from build123d import *

# Parameters (mm, degrees)
SKETCH1_R           = 20
SKETCH1_R_2         = 9.5
BOSS_EXTRUDE1_DEPTH = 55
SKETCH2_R           = 3.5
CUT_EXTRUDE1_DEPTH  = 12.66666667


with BuildPart() as part:
    # Sketch1 → Boss-Extrude1 (new body)
    with BuildSketch(Plane.XY):
        Circle(SKETCH1_R)
        Circle(SKETCH1_R_2, mode=Mode.SUBTRACT)
    extrude(amount=BOSS_EXTRUDE1_DEPTH)

    # Sketch2 → Cut-Extrude1 (cut, through all)
    with BuildSketch(Plane(origin=(8.33333333, 0, 0), x_dir=(0, 0, -1), z_dir=(1, 0, 0))):
        with Locations((-47.428775099, 14.493654617)):
            Circle(SKETCH2_R)
        with Locations((-7.571224901, -14.493654617)):
            Circle(SKETCH2_R)
    extrude(amount=CUT_EXTRUDE1_DEPTH, mode=Mode.SUBTRACT)


solid = part.part
Build history of the part. All positions in model axes, mm. A direction names the side the tool comes from. Give positions to 0.01 mm unless a question says otherwise; leave off trailing zeros. Write each loop counter-clockwise with the first axis right and the second up, starting at its lowest first coordinate (ties: lowest second). Pieces come first, ordered by that corner, then holes. Notation, with made-up numbers: (48.5, 13.25) - (75.5, 13.25) arc R24 cw to (75.5, 49.25) - close; hole circle Ø8 at (57, -32.5). An arc over 180 degrees is marked (long way). Use one line per item in the form item = value. Start each with the question number.
1. Probe line 1 (Y direction, x = 0, z = 37); line 2 (X direction, y = -0.5, z = 25); line 3 (Y direction, x = 4, z = 46). List the from-to ranges inside material, lowest first. Write a range as [from, to].
2. Band-saw the part on A-A on x = 0. Write the cut outline in (y, z), plus the area to 4 significant figures.
3. Drop flat-ended pins along their axis: pin 1 Ø8 at (x, y) = (12, -15.5) entering from -Z; pin 2 Ø10 at (x, z) = (-5.5, 20.5) entering from -Y; pin 3 Ø3 at (x, z) = (-6, 10.5) entering from +Y; pin 4 Ø1 at (x, z) = (-8.5, 20) entering from -Y. Give the stop position or say it passes through.
4. 3-axis set-ups, long thin cutter, end or side, ignore diameter. For faces 5 (the face through (4, -9, 0)), 6 (the face through (8.333, 15, 47)): which of +Z, -Z, +X, -X, +Y, -Y reach the whole face in a straight line?
5. Band-saw the part on C-C on z = 34. Write the cut outline in (x, y), plus the area to 3 significant figures.
6. Band-saw the part on D-D on x = 12.5. Write the cut outline in (y, z).
7. Two-plate mould, pull along Y, no slides. Class faces 1 (the face through (-19.98, 0.88, 27.12)), 2 (the face through (4.38, -8.43, 27.12)), 3 (the face through (11.531, 11.077, 48.188)), 4 (the face through (4, -9, 55)): released by +Y, released by -Y, zero draft, split by the parting line, or undercut.
Conclusion:
q1.line_1 = [-20, -9.5], [9.5, 20]
q1.line_2 = [-19.99, -9.49], [9.49, 19.99]
q1.line_3 = [-19.6, -8.62], [8.62, 19.6]
q2.outline = (-20, 0) - (-9.5, 0) - (-9.5, 55) - (-20, 55) - close; (9.5, 0) - (20, 0) - (20, 55) - (9.5, 55) - close
q2.area = 1,155 mm²
q3.pin_1 = 0
q3.pin_2 = -19.99
q3.pin_3 = 19.49
q3.pin_4 = -18.33
q4.face_5 = -Z, +X, -X, +Y, -Y
q4.face_6 = +X
q5.outline = circle Ø40 at (0, 0); hole circle Ø19 at (0, 0)
q5.area = 973 mm²
q6.outline = (-15.61, 0) - (15.61, 0) - (15.61, 44.11) arc R3.5 cw (long way) to (15.61, 50.75) - (15.61, 55) - (-15.61, 55) - (-15.61, 10.89) arc R3.5 cw (long way) to (-15.61, 4.25) - close
q7.face_1 = split by the parting line
q7.face_2 = undercut
q7.face_3 = undercut
q7.face_4 = zero draft
